The model under review builds one solid part; all positions refer to its coordinate system, in mm. Give positions to 0.01 mm unless a question says otherwise; leave off trailing zeros. Write each loop counter-clockwise with the first axis right and the second up, starting at its lowest first coordinate (ties: lowest second). Pieces come first, ordered by that corner, then holes. Notation, with made-up numbers: (58, 33.5) - (115, 33.5) arc R15 cw to (115, 62.5) - close; hole circle Ø2 at (33, 31.5). An arc over 180 degrees is marked (long way). One line per question, with ' | ' between items. Start each with the question number.
```python
from build123d import *

# Parameters (mm, degrees)
F0_R     = 5.5
F0_R_2   = 2.5
F1_DEPTH = 8
F2_R     = 2
F3_DEPTH = 6
F4_SIZE  = 1


with BuildPart() as f1:
    # F0 (on Top) → F1 (new body)
    with BuildSketch(Plane.XY):
        Circle(F0_R)
        Circle(F0_R_2, mode=Mode.SUBTRACT)
        Circle(F0_R_2)
    extrude(amount=F1_DEPTH)

    # F2
    f2_edges = [f1.edges().sort_by_distance(p)[0] for p in [
        (-5.5, 0, 8),
    ]]
    fillet(f2_edges, radius=F2_R)

    # F0 (on Top) → F3 (cut)
    with BuildSketch(Plane.XY):
        Circle(F0_R_2)
    extrude(amount=F3_DEPTH, mode=Mode.SUBTRACT)

    # F4
    f4_edges = [f1.edges().sort_by_distance(p)[0] for p in [
        (-5.5, 0, 0),
    ]]
    chamfer(f4_edges, length=F4_SIZE)


solid = f1.part
```
Item 1: Clearance check with flat-ended pins moving along their axes: P1, Ø4.5, axis at x = 0, y = 0, coming from the -Z side; P2, Ø4, axis at y = 2.5, z = 1, coming from the -X side; P3, Ø3, axis at y = -2, z = 6.5, coming from the +X side. State where each tip first meets the part, or that it passes through.
Item 2: Take a section at A-A (z = 4.5). Give the boundary of the cut face in (x, y), plus the area to 3 significant figures.
Item 3: For probe 1 along Y at (x, z) = (0, 2.4); probe 2 along Z at (x, y) = (2, 0.5); probe 3 along Y at (x, z) = (0.5, 2.5), list the stretches that pass through material, from the lowest coordinate up.
Item 4: Take a section at B-B (x = 0). Give the boundary of the cut face in (y, z).
Item 5: Take a section at C-C (z = 0.75). Give the boundary of the cut face in (x, y), plus the area to 3 significant figures.
Item 6: The part is to be moulded in two halves that separate along Y. For faces 1 (the flat face through (2, -2, 0)), 2 (the flat face through (0, 0, 6)), 3 (the cylindrical face through (-1.19, -5.37, 3.46)), 4 (the cylindrical face through (-0.54, -2.44, 2.96)), say which applies: +Y half, -Y half, draft (parallel to the pull), parting line (faces both ways), or undercut.
Check sheet entries:
1) P1: stops at z = 6 | P2: stops at x = -5.48 | P3: stops at x = 5.47
2) outline: circle Ø11 at (0, 0); hole circle Ø5 at (0, 0) | area: 75.4 mm^2
3) probe 1: y = -5.5 to -2.5, 2.5 to 5.5 | probe 2: z = 6 to 8 | probe 3: y = -5.48 to -2.45, 2.45 to 5.48
4) outline: (-5.5, 1) - (-4.5, 0) - (-2.5, 0) - (-2.5, 6) - (2.5, 6) - (2.5, 0) - (4.5, 0) - (5.5, 1) - (5.5, 6) arc R2 ccw to (3.5, 8) - (-3.5, 8) arc R2 ccw to (-5.5, 6) - close
5) outline: circle Ø10.5 at (0, 0); hole circle Ø5 at (0, 0) | area: 67.0 mm^2
6) face 1: draft | face 2: undercut | face 3: parting line | face 4: undercut
